from build123d import *

# Parameters (mm, degrees)
CROQUIS1_W              = 42
CROQUIS1_H              = 20
SALIENTE_EXTRUIR1_DEPTH = 90
CROQUIS2_R              = 1.75
CORTAR_EXTRUIR1_DEPTH   = 3
REDONDEO1_R             = 5
REDONDEO2_R             = 5


with BuildPart() as part:
    # Croquis1 → Saliente-Extruir1 (new body)
    with BuildSketch(Plane.XY):
        with Locations((21, -10)):
            Rectangle(CROQUIS1_W, CROQUIS1_H)
    extrude(amount=SALIENTE_EXTRUIR1_DEPTH)

    # Croquis2 → Cortar-Extruir1 (cut)
    with BuildSketch(Plane.XZ.offset(20)):
        with Locations(Location((8.5, 62, 0), (0, 0, 270))):
            Circle(CROQUIS2_R)
        with Locations(Location((33.5, 62, 0), (0, 0, 270))):
            Circle(CROQUIS2_R)
        with Locations(Location((33.5, 28, 0), (0, 0, 90))):
            Circle(CROQUIS2_R)
        with Locations(Location((8.5, 28, 0), (0, 0, 90))):
            Circle(CROQUIS2_R)
    extrude(amount=-CORTAR_EXTRUIR1_DEPTH, mode=Mode.SUBTRACT)

    # Redondeo1
    redondeo1_edges = [part.edges().sort_by_distance(p)[0] for p in [
        (42, 0, 45),
    ]]
    fillet(redondeo1_edges, radius=REDONDEO1_R)

    # Redondeo2
    redondeo2_edges = [part.edges().sort_by_distance(p)[0] for p in [
        (0, 0, 45),
    ]]
    fillet(redondeo2_edges, radius=REDONDEO2_R)


solid = part.part
Part model, mm, in its own coordinate system. A direction names the side the tool comes from. Round coordinates to 2 decimals unless told otherwise and drop trailing zeros. Write each loop counter-clockwise with the first axis right and the second up, starting at its lowest first coordinate (ties: lowest second). Pieces come first, ordered by that corner, then holes. Notation, with made-up numbers: M -20,3 L 23,3 A26 ccw 23,18 Z; hole C 87,28 d1. An arc over 180 degrees is marked long. Return JSON: item names as keys, results as strings. Group by question number.
(1) Pin check, flat tips, straight feed: pin 1 Ø4 at (x, z) = (34, 61.5) entering from -Y; pin 2 Ø1 at (x, z) = (8.5, 62) entering from -Y. Stop position of each tip, or through.
(2) Drill centre lines: probe 1 along X at (y, z) = (-19.3, 62); probe 2 along Y at (x, z) = (34, 62); probe 3 along Y at (x, z) = (4, 57). Where is each one in solid material? Low to high.
(3) Saw through at A-A on z = 62. Write the cut outline in (x, y).
(4) Two-plate mould, pull along Z, no slides. Class faces 1 (the face through (33.42, -18.52, 26.25)), 2 (the face through (42, -13, 44)), 3 (the face through (21, -10, 90)): +Z half, -Z half, draft (parallel to the pull), parting line (faces both ways), or undercut.
(5) Saw through at B-B on y = -1.25. Write the cut outline in (x, z).
(6) Which spindle directions (+Z, -Z, +X, -X, +Y, -Y) get a long thin tool onto all of the face, cutting with end or side? Do faces 4 (the face through (2, -1, 46)), 5 (the face through (8.42, -18.52, 26.25)). Say none if no direction does.
Returned:
{
 "1": {"pin 1": "y = -20", "pin 2": "y = -17"},
 "2": {"probe 1": "0 to 6.75, 10.25 to 31.75, 35.25 to 42", "probe 2": "-17 to 0", "probe 3": "-20 to -0.1"},
 "3": {"outline": "M 0,-20 L 6.75,-20 L 6.75,-17 L 10.25,-17 L 10.25,-20 L 31.75,-20 L 31.75,-17 L 35.25,-17 L 35.25,-20 L 42,-20 L 42,-5 A5 ccw 37,0 L 5,0 A5 ccw 0,-5 Z"},
 "4": {"face 1": "undercut", "face 2": "draft", "face 3": "+Z half"},
 "5": {"outline": "M 1.69,0 L 40.31,0 L 40.31,90 L 1.69,90 Z"},
 "6": {"face 4": "+Z, -Z, -X, +Y", "face 5": "-Y"}
}
